Model file for the job. Use its own axes, mm. Face numbers are marked on the shaded views. A direction names the side the tool comes from. Coordinates: 2 decimals unless noted, no trailing zeros. Order: outer loops, then holes, each group sorted by start corner. A loop starts at its lowest first (then second) coordinate and runs counter-clockwise, first axis right, second up. Notation, with made-up numbers: (56.5, 19.25) -> (101.5, 19.25) arc R18 cw to (101.5, 40.25) -> close; hole circle Ø3 at (13, -28). An arc over 180 degrees is marked (long way). Write item = value, one per line. Start each with the question number.
Q1. Cut at B-B, the plane x = -4.5. List the corners of the cut face in (y, z), plus the area to 3 significant figures.
Q2. Wall check: line 1 (X direction, y = 2, z = -22); line 2 (Z direction, x = -18.5, y = 14); line 3 (X direction, y = 17.5, z = -2). Give the ranges that are in metal, low to high. Write a range as from..to.
Q3. Flat gauge pins, fed straight in: pin 1 (3 mm diameter, centred on x = -20.7, z = -22, fed in from +Y); pin 2 (5 mm diameter, centred on x = -11.5, y = 37, fed in from +Z); pin 3 (5 mm diameter, centred on x = 3.5, z = -35, fed in from +Y); pin 4 (5 mm diameter, centred on x = 0, y = 34, fed in from -Z). Where does each tip first touch, or does it go through?
Q4. 3-axis set-ups, long thin cutter, end or side, ignore diameter. For the marked faces 1 and 2: which of +Z, -Z, +X, -X, +Y, -Y reach the whole face in a straight line?
Q5. Cut at C-C, the plane y = 25.5. List the corners of the cut face in (x, z), plus the area to 3 significant figures.
Q6. Cut at A-A, the plane z = -22. List the corners of the cut face in (x, y).
Q7. Cut at D-D, the plane x = 7. List the corners of the cut face in (y, z), plus the area to 3 significant figures.
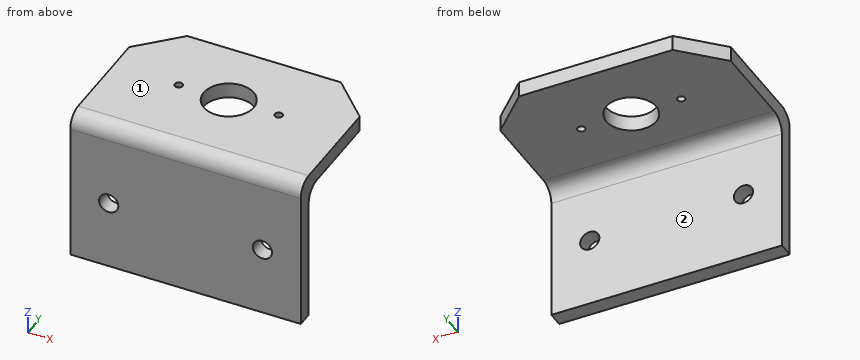
Autodesk Inventor part; units mm, degrees
ref_plane "YZ Plane" through (0, 0, 0) normal (1, 0, 0) x (0, 1, 0)
ref_plane "XZ Plane" through (0, 0, 0) normal (0, 1, 0) x (-1, 0, 0)
ref_plane "XY Plane" through (0, 0, 0) normal (0, 0, 1) x (1, 0, 0)
sketch "Sketch1" plane through (0, 0, 0) normal (0, 0, 1) x (1, 0, 0)
  line L0 (-30.7007, 0.9343) -> (29.2993, 0.9343)
  line L1 (-30.7007, 0.9343) -> (29.2993, 0.9343) construction
  line L2 (29.2993, 0.9343) -> (29.2993, 30.9343)
  line L3 (-30.7007, 30.9343) -> (-30.7007, 0.9343)
  line L4 (-30.7007, 4.9343) -> (29.2993, 4.9343)
  line L5 (-30.7007, 30.9343) -> (-20.7007, 40.9343)
  line L6 (-30.7007, 30.9343) -> (-16.5586, 30.9343) construction
  line L7 (-0.7007, 4.9343) -> (-0.7007, 40.9093) construction
  circle A0 centre (-0.7007, 22.9218) radius 6.5
  line L8 (-0.7007, 22.9218) -> (29.2993, 22.9218) construction
  circle A1 centre (12.2993, 22.9218) radius 1
  line L9 (29.2993, 30.9343) -> (19.2993, 40.9343)
  line L10 (-20.7007, 40.9343) -> (19.2993, 40.9343)
  line L11 (-0.7007, 22.9218) -> (-30.7007, 22.9218) construction
  circle A2 centre (-13.7007, 22.9218) radius 1
  point P0 (-30.2757, 2.8287)
  dimension "d13" = 60
  dimension "d15" = 30
  dimension "d17" = 45
  dimension "d20" = 4
  dimension "d53" = 13
  dimension "d56" = 13
  dimension "d57" = 2
  dimension "d58" = 40
extrude "Extrusion3" add sketch "Sketch1" against normal blind 4 contours L3 L5 L10 L9 L2 L4
extrude "Extrusion4" add sketch "Sketch1" against normal blind 40 contours L3 L4 L2 L0
sketch "Sketch4" plane through (-30.7007, 4.9343, -4) normal (0, 1, 0) x (1, 0, 0)
  line L0 (60, 0) -> (60, 36)
  line L1 (60, 18) -> (0, 18) construction
  line L2 (0, 0) -> (0, 36)
  line L3 (0, 36) -> (60, 36)
  line L4 (30, 36) -> (30, 0) construction
  line L5 (10, 0) -> (50, 0)
  circle A0 centre (50, 18) radius 2.5
  circle A1 centre (10, 18) radius 2.5
  point P0 (30.7007, -4)
  dimension "d63" = 10
  dimension "d64" = 5
hole "Hole3" at (19.2993, 4.9343, -22) at (-20.7007, 4.9343, -22) direction (0, -1, 0) diameter 5 end through all
thread "Thread1"
thread "Thread2"
fillet "Fillet2" radius 4 1 edges at (-0.7007, 4.9343, -4)
fillet "Fillet3" radius 4 1 edges at (-0.7007, 0.9343, 0)
thread "Thread3"
thread "Thread4"
thread "Thread5"
thread "Thread6"
properties part number "MotorHolder" material "Steel, Alloy"
Here are the results:
q1.outline = (0.93, -40) -> (4.93, -40) -> (4.93, -8) arc R4 cw to (8.93, -4) -> (17.65, -4) -> (17.65, 0) -> (4.93, 0) arc R4 ccw to (0.93, -4) -> close; (28.2, -4) -> (40.93, -4) -> (40.93, 0) -> (28.2, 0) -> close
q1.area = 262 mm²
q2.line_1 = -30.7..-23.2, -18.2..16.8, 21.8..29.3
q2.line_2 = -4..0
q2.line_3 = -30.7..-4.29, 2.88..29.3
q3.pin_1 = through
q3.pin_2 = 0
q3.pin_3 = 4.93
q3.pin_4 = -4
q4.face_1 = +Z, +X, -X, +Y, -Y
q4.face_2 = -Z, +X, -X, +Y
q5.outline = (-30.7, -4) -> (-6.67, -4) -> (-6.67, 0) -> (-30.7, 0) -> close; (5.27, -4) -> (29.3, -4) -> (29.3, 0) -> (5.27, 0) -> close
q5.area = 192 mm²
q6.outline = (-30.7, 0.93) -> (-23.2, 0.93) -> (-23.2, 4.93) -> (-30.7, 4.93) -> close; (-18.2, 0.93) -> (16.8, 0.93) -> (16.8, 4.93) -> (-18.2, 4.93) -> close; (21.8, 0.93) -> (29.3, 0.93) -> (29.3, 4.93) -> (21.8, 4.93) -> close
q7.outline = (0.93, -40) -> (4.93, -40) -> (4.93, -8) arc R4 cw to (8.93, -4) -> (40.93, -4) -> (40.93, 0) -> (4.93, 0) arc R4 ccw to (0.93, -4) -> close
q7.area = 304 mm²
